The model under review builds one solid part; all positions refer to its coordinate system, in mm. Face numbers are marked on the shaded views. A direction names the side the tool comes from. Round coordinates to 2 decimals unless told otherwise and drop trailing zeros. Write each loop counter-clockwise with the first axis right and the second up, starting at its lowest first coordinate (ties: lowest second). Pieces come first, ordered by that corner, then holes. Notation, with made-up numbers: (87, 51) - (134, 51) arc R12 ccw to (134, 59) - close; hole circle Ø3 at (-31, 88). An arc over 180 degrees is marked (long way). Use one line per item in the form item = value.
from build123d import *

# Parameters (mm, degrees)
CROQUIS1_W                 = 54
CROQUIS1_H                 = 50.3
CROQUIS1_W_2               = 50
CROQUIS1_H_2               = 46.3
SALIENTE_EXTRUIR1_DEPTH    = 24
CROQUIS2_W                 = 54
CROQUIS2_H                 = 50.3
SALIENTE_EXTRUIR2_DEPTH    = 2
CORTAR_EXTRUIR4_DEPTH      = 54
CORTAR_EXTRUIR5_REACH      = 75.646
CROQUIS7_W                 = 5.111111111
CROQUIS7_H                 = 42.3
CROQUIS7_W_2               = 5.111111112
CORTAR_EXTRUIR6_DEPTH      = 59.725548103
CORTAR_EXTRUIR6_DEPTH_BACK = 59.725548103
CROQUIS8_R                 = 6.35


with BuildPart() as part:
    # Croquis1 → Saliente-Extruir1 (new body)
    with BuildSketch(Plane(origin=(0, 0, 0), x_dir=(1, 0, 0), z_dir=(0, 1, 0))):
        with Locations((-25, -23.15)):
            Rectangle(CROQUIS1_W, CROQUIS1_H)
        with Locations((-25, -23.15)):
            Rectangle(CROQUIS1_W_2, CROQUIS1_H_2, mode=Mode.SUBTRACT)
    extrude(amount=SALIENTE_EXTRUIR1_DEPTH)

    # Croquis2 → Saliente-Extruir2 (add)
    with BuildSketch(Plane.XZ):
        with Locations((-25, 23.15)):
            Rectangle(CROQUIS2_W, CROQUIS2_H)
    extrude(amount=SALIENTE_EXTRUIR2_DEPTH)

    # Croquis6 → Cortar-Extruir4 (cut)
    with BuildSketch(Plane.ZY.offset(52)):
        Polygon((46.3, 24), (46.3, 0), (46.3, -2), (48.3, -2), (48.3, 24), align=None)
    extrude(amount=-CORTAR_EXTRUIR4_DEPTH, mode=Mode.SUBTRACT)

    # Croquis7 → Cortar-Extruir5 (cut, up to next)
    with BuildSketch(Plane(origin=(0, 0, 0), x_dir=(1, 0, 0), z_dir=(0, 1, 0)), mode=Mode.PRIVATE) as cortar_extruir5_sk1:
        with Locations((-45.444444445, -23.15)):
            Rectangle(CROQUIS7_W, CROQUIS7_H)
    cortar_extruir5_tool1 = extrude(cortar_extruir5_sk1.sketch, amount=-CORTAR_EXTRUIR5_REACH, mode=Mode.PRIVATE) & part.part
    # Croquis7 → Cortar-Extruir5 (cut, up to next)
    with BuildSketch(Plane(origin=(0, 0, 0), x_dir=(1, 0, 0), z_dir=(0, 1, 0)), mode=Mode.PRIVATE) as cortar_extruir5_sk2:
        with Locations((-35.222222223, -23.15)):
            Rectangle(CROQUIS7_W, CROQUIS7_H)
    cortar_extruir5_tool2 = extrude(cortar_extruir5_sk2.sketch, amount=-CORTAR_EXTRUIR5_REACH, mode=Mode.PRIVATE) & part.part
    # Croquis7 → Cortar-Extruir5 (cut, up to next)
    with BuildSketch(Plane(origin=(0, 0, 0), x_dir=(1, 0, 0), z_dir=(0, 1, 0)), mode=Mode.PRIVATE) as cortar_extruir5_sk3:
        with Locations((-14.777777778, -23.15)):
            Rectangle(CROQUIS7_W, CROQUIS7_H)
    cortar_extruir5_tool3 = extrude(cortar_extruir5_sk3.sketch, amount=-CORTAR_EXTRUIR5_REACH, mode=Mode.PRIVATE) & part.part
    # Croquis7 → Cortar-Extruir5 (cut, up to next)
    with BuildSketch(Plane(origin=(0, 0, 0), x_dir=(1, 0, 0), z_dir=(0, 1, 0)), mode=Mode.PRIVATE) as cortar_extruir5_sk4:
        with Locations((-4.555555555, -23.15)):
            Rectangle(CROQUIS7_W, CROQUIS7_H)
    cortar_extruir5_tool4 = extrude(cortar_extruir5_sk4.sketch, amount=-CORTAR_EXTRUIR5_REACH, mode=Mode.PRIVATE) & part.part
    # Croquis7 → Cortar-Extruir5 (cut, up to next)
    with BuildSketch(Plane(origin=(0, 0, 0), x_dir=(1, 0, 0), z_dir=(0, 1, 0)), mode=Mode.PRIVATE) as cortar_extruir5_sk5:
        with Locations((-25, -23.15)):
            Rectangle(CROQUIS7_W_2, CROQUIS7_H)
    cortar_extruir5_tool5 = extrude(cortar_extruir5_sk5.sketch, amount=-CORTAR_EXTRUIR5_REACH, mode=Mode.PRIVATE) & part.part
    add(cortar_extruir5_tool1.solids().sort_by_distance((-45.444444, 0, 23.15))[0], mode=Mode.SUBTRACT)
    add(cortar_extruir5_tool2.solids().sort_by_distance((-35.222222, 0, 23.15))[0], mode=Mode.SUBTRACT)
    add(cortar_extruir5_tool3.solids().sort_by_distance((-14.777778, 0, 23.15))[0], mode=Mode.SUBTRACT)
    add(cortar_extruir5_tool4.solids().sort_by_distance((-4.555556, 0, 23.15))[0], mode=Mode.SUBTRACT)
    add(cortar_extruir5_tool5.solids().sort_by_distance((-25, 0, 23.15))[0], mode=Mode.SUBTRACT)

    # Croquis8 → Cortar-Extruir6 (cut, two sides: drawn at the far end of the back side and taken through both)
    with BuildSketch(Plane(origin=(-25, 0, 0), x_dir=(0, 0, -1), z_dir=(1, 0, 0)).offset(-CORTAR_EXTRUIR6_DEPTH_BACK)):
        with Locations((-8, 15)):
            Circle(CROQUIS8_R)
    extrude(amount=CORTAR_EXTRUIR6_DEPTH + CORTAR_EXTRUIR6_DEPTH_BACK, mode=Mode.SUBTRACT)


solid = part.part
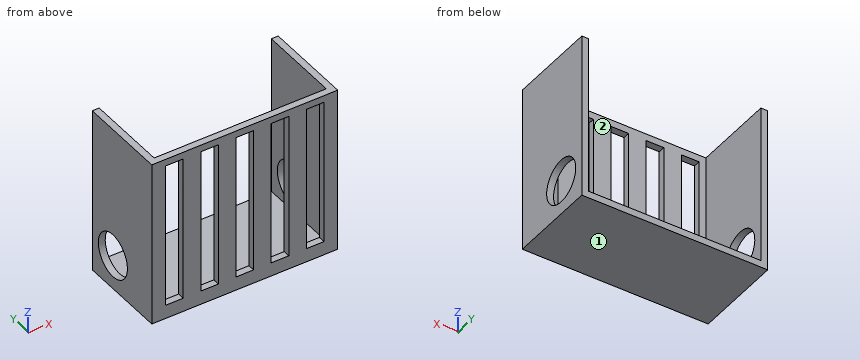
(1) To check wall thickness, follow L1, parallel to Y at x = -50.5, z = 8; L2, parallel to X at y = 18, z = 36; L3, parallel to Z at x = -50.8, y = 15. State the ranges of each line that lie inside material, in increasing order.
Geometry results:
L1 = -2 to 8.65, 21.35 to 24
L2 = -52 to -50, 0 to 2
L3 = -2 to 1.65, 14.35 to 46.3
(2) Add section C-C on x = -47. Write out the cut boundary in (y, z).
Geometry results:
outline = (-2, -2) - (24, -2) - (24, 0) - (0, 0) - (0, 2) - (-2, 2) - close; (-2, 44.3) - (0, 44.3) - (0, 46.3) - (-2, 46.3) - close
(3) Add section A-A on z = 37.5. Write out the cut boundary in (x, y).
Geometry results:
outline = (-52, -2) - (-48, -2) - (-48, 0) - (-50, 0) - (-50, 24) - (-52, 24) - close; (-42.89, -2) - (-37.78, -2) - (-37.78, 0) - (-42.89, 0) - close; (-32.67, -2) - (-27.56, -2) - (-27.56, 0) - (-32.67, 0) - close; (-22.44, -2) - (-17.33, -2) - (-17.33, 0) - (-22.44, 0) - close; (-12.22, -2) - (-7.11, -2) - (-7.11, 0) - (-12.22, 0) - close; (-2, -2) - (2, -2) - (2, 24) - (0, 24) - (0, 0) - (-2, 0) - close
(4) Add section D-D on z = 1. Write out the cut boundary in (x, y).
Geometry results:
outline = (-52, -2) - (2, -2) - (2, 24) - (0, 24) - (0, 0) - (-50, 0) - (-50, 24) - (-52, 24) - close
(5) Add section B-B on y = 15. Write out the cut boundary in (x, z).
Geometry results:
outline = (-52, -2) - (2, -2) - (2, 1.65) - (0, 1.65) - (0, 0) - (-50, 0) - (-50, 1.65) - (-52, 1.65) - close; (-52, 14.35) - (-50, 14.35) - (-50, 46.3) - (-52, 46.3) - close; (0, 14.35) - (2, 14.35) - (2, 46.3) - (0, 46.3) - close
(6) Insertion check: P1, Ø1, axis at x = -22, y = 20, coming from the +Z side; P2, Ø23, axis at x = -21, z = 29.5, coming from the +Y side; P3, Ø10, axis at x = -46.5, z = 35, coming from the +Y side. Each pin has a flat end and moves straight along its axis. Give the tip position at first contact, or say it passes through.
Geometry results:
P1 = 0
P2 = 0
P3 = 24
(7) Machinability: for the marked faces 1 and 2, which of the approach directions +Z, -Z, +X, -X, +Y, -Y give a long, thin tool a straight path to every point of the face, cutting with its end or side? Answer none if there is none.
Geometry results:
face_1 = -Z, +X, -X, +Y, -Y
face_2 = +Z, +Y
